Build history of the part. All positions in model axes, mm. Coordinates: 2 decimals unless noted, no trailing zeros. Order: outer loops, then holes, each group sorted by start corner. A loop starts at its lowest first (then second) coordinate and runs counter-clockwise, first axis right, second up. Notation, with made-up numbers: (73, 45) - (129, 45) arc R22 ccw to (129, 82) - close; hole circle Ø5 at (-4, 49). An arc over 180 degrees is marked (long way). Return JSON: item names as keys, results as strings.
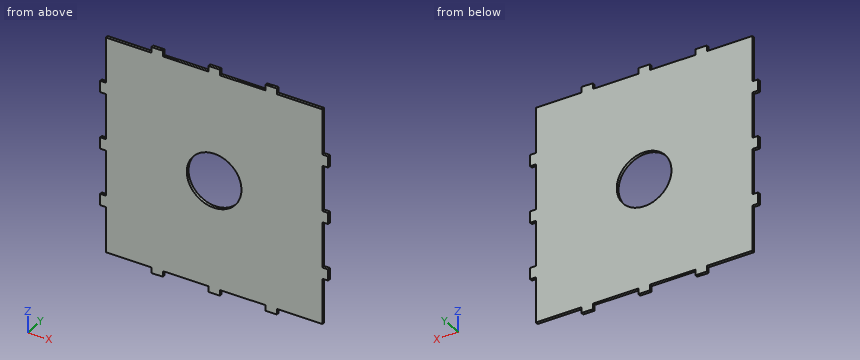
from build123d import *

# Parameters (mm, degrees)
SKETCH1_R           = 15.24
BOSS_EXTRUDE1_DEPTH = 1.5875


with BuildPart() as part:
    # Sketch1 → Boss-Extrude1 (new body)
    with BuildSketch(Plane(origin=(0, 0, 0), x_dir=(1, 0, 0), z_dir=(0, 1, 0))):
        Polygon((3.175, 63.5), (-3.175, 63.5), (-3.175, 60.325), (-28.575, 60.325), (-28.575, 63.5), (-34.925, 63.5), (-34.925, 60.325), (-60.325, 60.325), (-60.325, 34.925), (-63.5, 34.925), (-63.5, 28.575), (-60.325, 28.575), (-60.325, 3.175), (-63.5, 3.175), (-63.5, -3.175), (-60.325, -3.175), (-60.325, -28.575), (-63.5, -28.575), (-63.5, -34.925), (-60.325, -34.925), (-60.325, -60.325), (-34.925, -60.325), (-34.925, -63.5), (-28.575, -63.5), (-28.575, -60.325), (-3.175, -60.325), (-3.175, -63.5), (3.175, -63.5), (3.175, -60.325), (28.575, -60.325), (28.575, -63.5), (34.925, -63.5), (34.925, -60.325), (60.325, -60.325), (60.325, -34.925), (63.5, -34.925), (63.5, -28.575), (60.325, -28.575), (60.325, -3.175), (63.5, -3.175), (63.5, 3.175), (60.325, 3.175), (60.325, 28.575), (63.5, 28.575), (63.5, 34.925), (60.325, 34.925), (60.325, 60.325), (34.925, 60.325), (34.925, 63.5), (28.575, 63.5), (28.575, 60.325), (3.175, 60.325), align=None)
        with Locations(Location((0, 0, 0), (0, 0, 270))):
            Circle(SKETCH1_R, mode=Mode.SUBTRACT)
    extrude(amount=BOSS_EXTRUDE1_DEPTH)


solid = part.part
1. Drop flat-ended pins along their axis: pin 1 (0.8 mm diameter, centred on x = 62.5, y = 0.5, fed in from +Z) (3 decimals); pin 2 (4 mm diameter, centred on x = 9.5, z = -46, fed in from -Y); pin 3 (0.5 mm diameter, centred on y = 0.5, z = -61.5, fed in from +X) (3 decimals); pin 4 (0.8 mm diameter, centred on x = 62, y = 1, fed in from -Z) (3 decimals). Give the stop position or say it passes through.
Check values:
{"pin 1": "z = 34.925", "pin 2": "y = 0", "pin 3": "x = 34.925", "pin 4": "z = -34.925"}
2. Probe L1, parallel to X at y = 0.4, z = -0.5; L2, parallel to Z at x = -1, y = 0.9; L3, parallel to Z at x = -53, y = 0.45 (3 decimals). List the from-to ranges inside material, lowest first.
Check values:
{"L1": "-63.5 to -15.23, 15.23 to 63.5", "L2": "-63.5 to -15.21, 15.21 to 63.5", "L3": "-60.325 to 60.325"}
3. Cut at D-D on x = -17. Give the cut face in (y, z) (1 decimal), plus the area to 3 significant figures.
Check values:
{"outline": "(0, -60.3) - (1.6, -60.3) - (1.6, 60.3) - (0, 60.3) - close", "area": "192 mm²"}
4. Cut at B-B on z = 0. Give the cut face in (x, y).
Check values:
{"outline": "(-63.5, 0) - (-15.24, 0) - (-15.24, 1.59) - (-63.5, 1.59) - close; (15.24, 0) - (63.5, 0) - (63.5, 1.59) - (15.24, 1.59) - close"}
5. Cut at C-C on z = -17.5. Give the cut face in (x, y) (1 decimal).
Check values:
{"outline": "(-60.3, 0) - (60.3, 0) - (60.3, 1.6) - (-60.3, 1.6) - close"}
6. Cut at A-A on x = 0. Give the cut face in (y, z).
Check values:
{"outline": "(0, -63.5) - (1.59, -63.5) - (1.59, -15.24) - (0, -15.24) - close; (0, 15.24) - (1.59, 15.24) - (1.59, 63.5) - (0, 63.5) - close"}
